Input: part model. Units: mm. Frame: model coordinates. A direction names the side the tool comes from. Coordinates: 2 decimals unless noted, no trailing zeros. Loops run counter-clockwise (first coordinate to the right, second up) from the corner with the lowest first, then second, coordinate; pieces in that order, holes last.
```python
from build123d import *

# Parameters (mm, degrees)
SKETCH_2_R               = 5
EXTRUDE_1_DEPTH          = 5
SKETCH_3_R               = 12
EXTRUDE_2_DEPTH          = 2
SKETCH_5_R               = 3.5
SKETCH_5_R_2             = 1.5
EXTRUDE_3_DEPTH          = 12
EXTRUDE_4_DEPTH          = 15
PATTERN_CIRCULAR_1_COUNT = 5
CUT_EXTRUDE_START        = -15
CUT_EXTRUDE_1_DEPTH      = 15
PATTERN_CIRCULAR_2_COUNT = 5


with BuildPart() as part:
    # 草图1 → 旋转1 (revolve)
    with BuildSketch(Plane.XY, mode=Mode.PRIVATE) as revolve_1_sk:
        with BuildLine():
            Line((19.5, 9.5), (19.5, -7.5))
            Line((19.5, -7.5), (0, -7.5))
            Line((0, -7.5), (0, -9.5))
            Line((0, -9.5), (21.75, -9.5))
            ThreePointArc((21.75, -9.5), (23.164213562, -8.914213562), (23.75, -7.5))
            Line((23.75, -7.5), (23.75, 7.5))
            ThreePointArc((23.75, 7.5), (23.164213562, 8.914213562), (21.75, 9.5))
            Line((21.75, 9.5), (19.5, 9.5))
        make_face()
    revolve(revolve_1_sk.sketch.rotate(Axis((0, 0, 0), (0, -1, 0)), 90), axis=Axis((0, 0, 0), (0, -1, 0)))

    # 草图2 → 凸台-拉伸1 (add)
    with BuildSketch(Plane(origin=(0, -7.5, 0), x_dir=(1, 0, 0), z_dir=(0, 1, 0))):
        with Locations(Location((0, 0, 0), (0, 0, 90))):
            Circle(SKETCH_2_R)
    extrude(amount=EXTRUDE_1_DEPTH)

    # 草图3 → 凸台-拉伸2 (add)
    with BuildSketch(Plane(origin=(0, -2.5, 0), x_dir=(1, 0, 0), z_dir=(0, 1, 0))):
        with Locations(Location((0, 0, 0), (0, 0, 270))):
            Circle(SKETCH_3_R)
    extrude(amount=EXTRUDE_2_DEPTH)

    # 草图5 → 凸台-拉伸3 (add)
    with BuildSketch(Plane(origin=(0, -0.5, 0), x_dir=(1, 0, 0), z_dir=(0, 1, 0))):
        with Locations(Location((0, 0, 0), (0, 0, 270))):
            Circle(SKETCH_5_R)
        with Locations(Location((0, 0, 0), (0, 0, 270))):
            Circle(SKETCH_5_R_2, mode=Mode.SUBTRACT)
    extrude(amount=EXTRUDE_3_DEPTH)

    # 草图6 → 凸台-拉伸4 (add)
    with BuildSketch(Plane(origin=(0, -7.5, 0), x_dir=(1, 0, 0), z_dir=(0, 1, 0))):
        with BuildLine():
            Line((-0.5, 19.49358869), (-0.5, 3.464101615))
            ThreePointArc((-0.5, 3.464101615), (0, 3.5), (0.5, 3.464101615))
            Line((0.5, 3.464101615), (0.5, 19.49358869))
            ThreePointArc((0.5, 19.49358869), (0, 19.5), (-0.5, 19.49358869))
        make_face()
    extrude_4 = extrude(amount=EXTRUDE_4_DEPTH)

    # 阵列(圆周)1: 凸台-拉伸4 ×5 about axis
    pattern_circular_1_axis = Axis((0, 0, 0), (0, 1, 0))
    for i in range(1, PATTERN_CIRCULAR_1_COUNT):
        add(extrude_4.rotate(pattern_circular_1_axis, i * 360 / PATTERN_CIRCULAR_1_COUNT))

    # 草图7 → 切除-拉伸1 (cut)
    with BuildSketch(Plane(origin=(0, -7.5, 0), x_dir=(1, 0, 0), z_dir=(0, 1, 0)).offset(CUT_EXTRUDE_START)):
        with BuildLine():
            Line((1.254341559, 11.934262744), (1.567926949, 14.917828431))
            ThreePointArc((1.567926949, 14.917828431), (8.816778784, 12.135254916), (13.703181865, 6.101049646))
            Line((13.703181865, 6.101049646), (10.962545492, 4.880839717))
            ThreePointArc((10.962545492, 4.880839717), (7.053423028, 9.708203932), (1.254341559, 11.934262744))
        make_face()
    cut_extrude_1 = extrude(amount=CUT_EXTRUDE_1_DEPTH, mode=Mode.SUBTRACT)

    # 阵列(圆周)2: 切除-拉伸1 ×5 about axis
    pattern_circular_2_axis = Axis((0, 0, 0), (0, 1, 0))
    for i in range(1, PATTERN_CIRCULAR_2_COUNT):
        add(cut_extrude_1.rotate(pattern_circular_2_axis, i * 360 / PATTERN_CIRCULAR_2_COUNT), mode=Mode.SUBTRACT)


solid = part.part
```
Item 1: Section query B-B (z = 0). Count the separate pieces of the cut face and the enclosed holes in it, then the cut area to 3 significant figures.
Result:
separate pieces: 3
enclosed holes: 0
area: 370 mm2
Item 2: Section query C-C (y = -5). Output: boundary loops of the cut face in (x, z) (3 decimals), then the cut area to 3 significant figures.
Result:
outline: circle Ø47.5 at (0, 0); hole (-18.694, -5.548) - (-4.886, -1.062) arc R5 cw to (-3.329, 3.731) - (-11.863, 15.477) arc R19.5 ccw to start; hole (-18.385, -6.499) arc R19.5 ccw to (-0.5, -19.494) - (-0.5, -4.975) arc R5 cw to (-4.577, -2.013) - close; hole (-11.054, 16.065) - (-2.52, 4.319) arc R5 cw to (2.52, 4.319) - (11.054, 16.065) arc R19.5 ccw to start; hole (0.5, -19.494) arc R19.5 ccw to (18.385, -6.499) - (4.577, -2.013) arc R5 cw to (0.5, -4.975) - close; hole (3.329, 3.731) arc R5 cw to (4.886, -1.062) - (18.694, -5.548) arc R19.5 ccw to (11.863, 15.477) - close
area: 729 mm2
Item 3: Line query: L1, parallel to X at y = 3.5, z = 0; L2, parallel to X at y = -1, z = 0; L3, parallel to Y at x = -1.5, z = -10. Output: solid intervals per line, ascending.
Result:
L1: x = -23.75 to -19.5, -3.5 to -1.5, 1.5 to 3.5, 19.5 to 23.75
L2: x = -23.75 to -19.5, -12 to 12, 19.5 to 23.75
L3: y = -9.5 to -7.5, -2.5 to -0.5
Item 4: Reachability of faces 1 (the face through (4.744, -5.035, 1.58)), 2 (the face through (1.05, 5.42, 3.34)), 3 (the face through (12.35, -8.51, -5.5)) from +Z, -Z, +X, -X, +Y, -Y: full face, straight path, thin tool, end or side. Return the list, or none.
Result:
face 1: none
face 2: +Y
face 3: +Y, -Y
Item 5: Contact query for flat-ended pins moving along their axis: P1, Ø10, axis at y = 4.5, z = 16.5, coming from the -X side; P2, Ø5, axis at x = 3, y = -3.5, coming from the +Z side; P3, Ø8.5, axis at x = 13.5, z = -8, coming from the +Y side. Output: stop coordinate, or through.
Result:
P1: stops at x = -20.78
P2: stops at z = 23.74
P3: stops at y = 9.5
Item 6: Section query A-A (y = 3.75). Output: boundary loops of the cut face in (x, z) (3 decimals).
Result:
outline: circle Ø47.5 at (0, 0); hole (-18.694, -5.548) - (-3.449, -0.595) arc R3.5 cw to (-2.441, 2.509) - (-11.863, 15.477) arc R19.5 ccw to start; hole (-18.385, -6.499) arc R19.5 ccw to (-0.5, -19.494) - (-0.5, -3.464) arc R3.5 cw to (-3.14, -1.546) - close; hole (-11.054, 16.065) - (-1.632, 3.096) arc R3.5 cw to (1.632, 3.096) - (11.054, 16.065) arc R19.5 ccw to start; hole circle Ø3 at (0, 0); hole (0.5, -19.494) arc R19.5 ccw to (18.385, -6.499) - (3.14, -1.546) arc R3.5 cw to (0.5, -3.464) - close; hole (2.441, 2.509) arc R3.5 cw to (3.449, -0.595) - (18.694, -5.548) arc R19.5 ccw to (11.863, 15.477) - close
Item 7: Mould query, pull axis X, two halves, no side actions, for faces 4 (the face through (-6.8, 7.5, 9.4)), 5 (the face through (0, 11.5, 2)). Classes: +X half, -X half, draft (parallel to the pull), parting line (faces both ways), or undercut.
Result:
face 4: undercut
face 5: draft
